The drawing under review shows one solid part. Ordinate dimensions are in mm from its lowest x, y, z. A direction names the side the tool comes from. Round coordinates to 2 decimals unless told otherwise and drop trailing zeros. Write each loop counter-clockwise with the first axis right and the second up, starting at its lowest first coordinate (ties: lowest second). Pieces come first, ordered by that corner, then holes. Notation, with made-up numbers: (-5, 49) - (53, 49) arc R13 ccw to (53, 69) - close; hole circle Ø3 at (86, -36). An arc over 180 degrees is marked (long way). Answer in a Markdown table with one row per item. Add a question column.
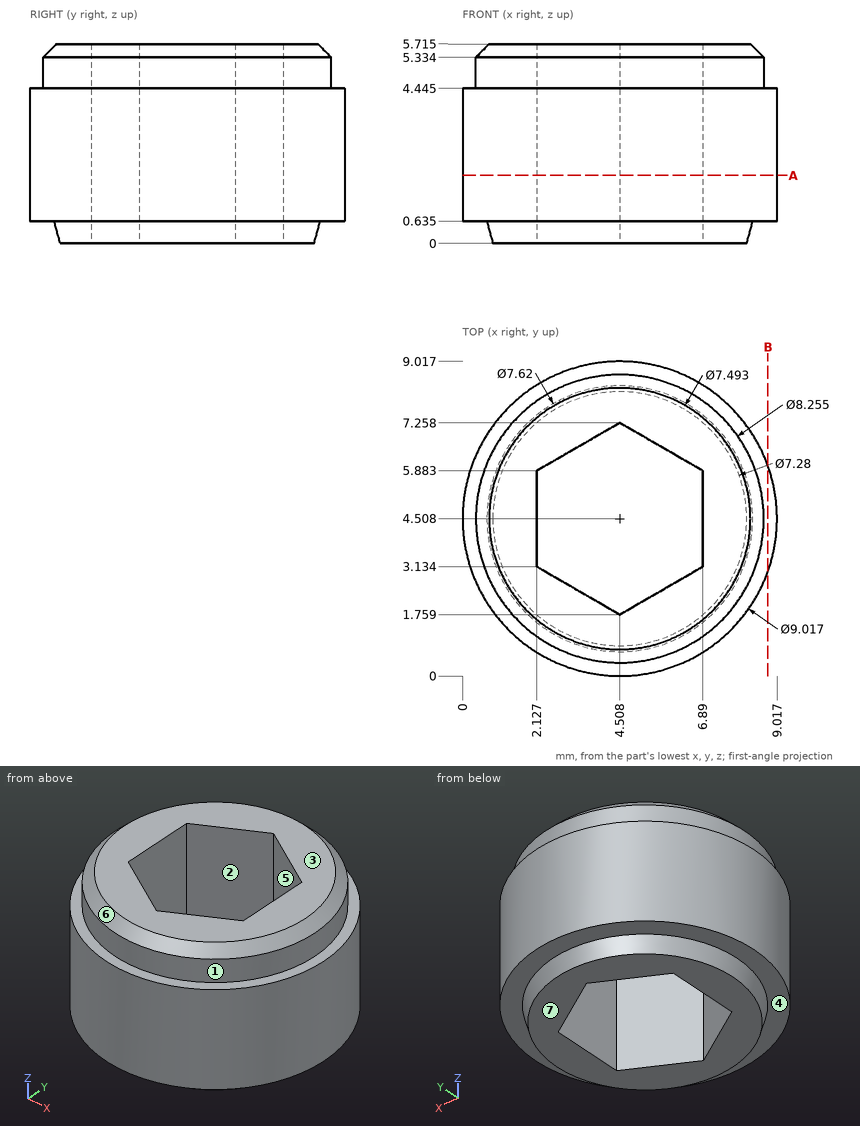
Q1. To check wall thickness, follow probe 1 along Y at (x, z) = (6.5, 1) (1 decimal); probe 2 along Y at (x, z) = (6, 5.4) (1 decimal); probe 3 along Z at (x, y) = (6.25, 0.5) (1 decimal). State the ranges of each line that lie inside material, in increasing order.
Q2. Draft analysis for pull direction Y (two halves, no side actions). For the marked faces 5, 6 and 7, state which applies: released by +Y, released by -Y, zero draft, split by the parting line, or undercut.
Q3. Insertion check: pin 1 Ø1.5 at (x, z) = (2, 4) entering from -Y; pin 2 Ø1 at (y, z) = (2, 2) entering from -X; pin 3 Ø1.5 at (x, y) = (1, 1.5) entering from -Z (1 decimal). Each pin has a flat end and moves straight along its axis. Give the tip position at first contact, or say it passes through.
Q4. Add section B-B on x = 8.75. State the section outline as (y, z) points (1 decimal).
Q5. Tool access review of the marked faces 1, 2, 3 and 4: name each direction out of +Z, -Z, +X, -X, +Y, -Y from which nothing blocks a thin tool from reaching the whole face with its end or side.
Q6. Add section A-A on z = 1.95. State the section outline as (x, y) points.
Answer sheet:
| question | item | result |
|---|---|---|
| 1 | probe 1 | y = 0.5 to 2.9, 6.1 to 8.6 |
| 1 | probe 2 | y = 0.7 to 2.6, 6.4 to 8.3 |
| 1 | probe 3 | z = 0.6 to 4.4 |
| 2 | face 5 | undercut |
| 2 | face 6 | split by the parting line |
| 2 | face 7 | zero draft |
| 3 | pin 1 | stops at y = 0.36 |
| 3 | pin 2 | stops at x = 0.47 |
| 3 | pin 3 | stops at z = 0.6 |
| 4 | outline | (3, 0.6) - (6, 0.6) - (6, 4.4) - (3, 4.4) - close |
| 5 | face 1 | +Z |
| 5 | face 2 | +Z, -Z |
| 5 | face 3 | +Z, +X, -X, +Y, -Y |
| 5 | face 4 | -Z |
| 6 | outline | circle Ø9.02 at (4.51, 4.51); hole (2.13, 3.13) - (4.51, 1.76) - (6.89, 3.13) - (6.89, 5.88) - (4.51, 7.26) - (2.13, 5.88) - close |
